Input: part model. Units: mm. Frame: model coordinates. A direction names the side the tool comes from. Coordinates: 2 decimals unless noted, no trailing zeros. Order: outer loops, then holes, each group sorted by start corner. A loop starts at its lowest first (then second) coordinate and runs counter-clockwise, first axis right, second up. Notation, with made-up numbers: (-6.75, 42) -> (35.25, 42) arc R25 cw to (35.25, 63) -> close; hole circle Ø1 at (-30, 3). An arc over 180 degrees is marked (long way). One line per question, with ' | ' between items.
```python
from build123d import *

# Parameters (mm, degrees)
SKETCH1_W           = 14.40065461
SKETCH1_H           = 29
SKETCH1_W_2         = 14
SKETCH1_R           = 1.35
BOSS_EXTRUDE2_DEPTH = 2
SKETCH2_R           = 7.5
CUT_EXTRUDE1_DEPTH  = 2
SKETCH3_W           = 5.497638463
SKETCH3_H           = 5.570940309
SKETCH3_W_2         = 9.162730771
SKETCH3_H_2         = 3.811696001
SKETCH3_W_3         = 6.450562463
SKETCH3_H_3         = 6.157355078
SKETCH3_W_4         = 5.570940309
SKETCH3_H_4         = 4.544714463
SKETCH3_W_5         = 6.27821864
SKETCH3_H_5         = 3.656250045
SKETCH3_W_6         = 6.338006476
SKETCH3_H_6         = 4.174139377
BOSS_EXTRUDE3_DEPTH = 2
SKETCH4_R           = 1.6
CUT_EXTRUDE2_DEPTH  = 10
CHAMFER1_SIZE       = 1
SKETCH5_W           = 10.813263603
SKETCH5_H           = 2.270321327
SKETCH5_W_2         = 10.386812418
SKETCH5_H_2         = 2.583327919
SKETCH5_W_3         = 10.884553744
SKETCH5_H_3         = 2.62287776
SKETCH5_W_4         = 12.051602383
SKETCH5_H_4         = 3.322696714
BOSS_EXTRUDE4_DEPTH = 2


with BuildPart() as part:
    # Sketch1 → Boss-Extrude2 (new body)
    with BuildSketch(Plane(origin=(0, 0, 0), x_dir=(1, 0, 0), z_dir=(0, 1, 0))):
        with Locations((-22.106428168, 0.106069008)):
            Rectangle(SKETCH1_W, SKETCH1_H)
        with Locations((21.693244527, 0.106069008)):
            Rectangle(SKETCH1_W_2, SKETCH1_H)
        with BuildLine():
            Line((22.693244527, -34.393930992), (26.693244527, -34.393930992))
            ThreePointArc((26.693244527, -34.393930992), (28.814564871, -33.515251336), (29.693244527, -31.393930992))
            Line((29.693244527, -31.393930992), (29.693244527, -24.393930992))
            Line((29.693244527, -24.393930992), (28.693244527, -24.393930992))
            Line((28.693244527, -24.393930992), (28.693244527, -14.393930992))
            Line((28.693244527, -14.393930992), (11.693244527, -14.393930992))
            Line((11.693244527, -14.393930992), (11.693244527, -26.393930992))
            Line((11.693244527, -26.393930992), (-12.306755473, -26.393930992))
            Line((-12.306755473, -26.393930992), (-12.306755473, -14.393930992))
            Line((-12.306755473, -14.393930992), (-29.306755473, -14.393930992))
            Line((-29.306755473, -14.393930992), (-29.306755473, -24.393930992))
            Line((-29.306755473, -24.393930992), (-30.306755473, -24.393930992))
            Line((-30.306755473, -24.393930992), (-30.306755473, -31.393930992))
            ThreePointArc((-30.306755473, -31.393930992), (-29.428075817, -33.515251336), (-27.306755473, -34.393930992))
            Line((-27.306755473, -34.393930992), (-25.306755473, -34.393930992))
            Line((-25.306755473, -34.393930992), (-25.306755473, -32.393930992))
            Line((-25.306755473, -32.393930992), (-15.306755473, -32.393930992))
            Line((-15.306755473, -32.393930992), (-15.306755473, -34.393930992))
            Line((-15.306755473, -34.393930992), (12.693244527, -34.393930992))
            Line((12.693244527, -34.393930992), (12.693244527, -32.393930992))
            Line((12.693244527, -32.393930992), (22.693244527, -32.393930992))
            Line((22.693244527, -32.393930992), (22.693244527, -34.393930992))
        make_face()
        with Locations((-20.98250428, -22.393930992)):
            Circle(SKETCH1_R, mode=Mode.SUBTRACT)
        with Locations((19.975772563, -22.393930992)):
            Circle(SKETCH1_R, mode=Mode.SUBTRACT)
        with Locations((-0.212217338, -28.393930992)):
            Circle(SKETCH1_R, mode=Mode.SUBTRACT)
        with BuildLine():
            Line((-23.306755473, 34.606069008), (-27.306755473, 34.606069008))
            ThreePointArc((-27.306755473, 34.606069008), (-29.428075817, 33.727389352), (-30.306755473, 31.606069008))
            Line((-30.306755473, 31.606069008), (-30.306755473, 24.606069008))
            Line((-30.306755473, 24.606069008), (-29.306755473, 24.606069008))
            Line((-29.306755473, 24.606069008), (-29.306755473, 14.606069008))
            Line((-29.306755473, 14.606069008), (28.693244527, 14.606069008))
            Line((28.693244527, 14.606069008), (28.693244527, 24.606069008))
            Line((28.693244527, 24.606069008), (29.693244527, 24.606069008))
            Line((29.693244527, 24.606069008), (29.693244527, 31.606069008))
            ThreePointArc((29.693244527, 31.606069008), (28.814564871, 33.727389352), (26.693244527, 34.606069008))
            Line((26.693244527, 34.606069008), (24.693244527, 34.606069008))
            Line((24.693244527, 34.606069008), (24.693244527, 32.606069008))
            Line((24.693244527, 32.606069008), (14.693244527, 32.606069008))
            Line((14.693244527, 32.606069008), (14.693244527, 34.606069008))
            Line((14.693244527, 34.606069008), (-13.306755473, 34.606069008))
            Line((-13.306755473, 34.606069008), (-13.306755473, 32.606069008))
            Line((-13.306755473, 32.606069008), (-23.306755473, 32.606069008))
            Line((-23.306755473, 32.606069008), (-23.306755473, 34.606069008))
        make_face()
        with Locations((-20.98250428, 22.606069008)):
            Circle(SKETCH1_R, mode=Mode.SUBTRACT)
        with Locations((-0.212217338, 28.606069008)):
            Circle(SKETCH1_R, mode=Mode.SUBTRACT)
        with Locations((19.975772563, 22.606069008)):
            Circle(SKETCH1_R, mode=Mode.SUBTRACT)
        with Locations((-0.212217338, 17.606069008)):
            Circle(SKETCH1_R, mode=Mode.SUBTRACT)
    extrude(amount=BOSS_EXTRUDE2_DEPTH)

    # Sketch2 → Cut-Extrude1 (cut)
    with BuildSketch(Plane(origin=(0, 2, 0), x_dir=(1, 0, 0), z_dir=(0, 1, 0))):
        with Locations((-0.212217338, 17.606069008)):
            Circle(SKETCH2_R)
    extrude(amount=-CUT_EXTRUDE1_DEPTH, mode=Mode.SUBTRACT)

    # Sketch3 → Boss-Extrude3 (add)
    with BuildSketch(Plane(origin=(0, 2, 0), x_dir=(1, 0, 0), z_dir=(0, 1, 0))):
        with Locations((-20.684668709, 22.829641321)):
            Rectangle(SKETCH3_W, SKETCH3_H)
        with Locations((0.426262988, 28.40058163)):
            Rectangle(SKETCH3_W_2, SKETCH3_H_2)
        with Locations((19.594695763, 21.950019167)):
            Rectangle(SKETCH3_W_3, SKETCH3_H_3)
        with Locations((20.03450684, -21.664579305)):
            Rectangle(SKETCH3_W_4, SKETCH3_H_4)
        with Locations((-1.015993077, -28.583465841)):
            Rectangle(SKETCH3_W_5, SKETCH3_H_5)
        with Locations((-20.264484702, -22.364159865)):
            Rectangle(SKETCH3_W_6, SKETCH3_H_6)
    extrude(amount=-BOSS_EXTRUDE3_DEPTH)

    # Sketch4 → Cut-Extrude2 (cut)
    with BuildSketch(Plane(origin=(0, 2, 0), x_dir=(1, 0, 0), z_dir=(0, 1, 0))):
        with BuildLine():
            ThreePointArc((-8.093244527, -27.893930992), (-8.379691654, -26.980378119), (-9.136468091, -26.393930992))
            Line((-9.136468091, -26.393930992), (-10.250020963, -26.393930992))
            ThreePointArc((-10.250020963, -26.393930992), (-10.6067974, -29.207483865), (-8.093244527, -27.893930992))
        make_face()
        with BuildLine():
            Line((-10.250020963, -26.393930992), (-9.136468091, -26.393930992))
            ThreePointArc((-9.136468091, -26.393930992), (-9.693244527, -26.293930992), (-10.250020963, -26.393930992))
        make_face()
        with Locations((-25.693244527, -27.893930992)):
            Circle(SKETCH4_R)
        with BuildLine():
            ThreePointArc((9.136468091, -26.393930992), (8.779691654, -29.207483865), (11.293244527, -27.893930992))
            ThreePointArc((11.293244527, -27.893930992), (11.0067974, -26.980378119), (10.250020963, -26.393930992))
            Line((10.250020963, -26.393930992), (9.136468091, -26.393930992))
        make_face()
        with BuildLine():
            Line((9.136468091, -26.393930992), (10.250020963, -26.393930992))
            ThreePointArc((10.250020963, -26.393930992), (9.693244527, -26.293930992), (9.136468091, -26.393930992))
        make_face()
        with Locations((25.693244527, -27.893930992)):
            Circle(SKETCH4_R)
        with Locations((25.693244527, 28.106069008)):
            Circle(SKETCH4_R)
        with Locations((9.693244527, 28.106069008)):
            Circle(SKETCH4_R)
        with Locations((-9.693244527, 28.106069008)):
            Circle(SKETCH4_R)
        with Locations((-25.693244527, 28.106069008)):
            Circle(SKETCH4_R)
    extrude(amount=-CUT_EXTRUDE2_DEPTH, mode=Mode.SUBTRACT)

    # Chamfer1
    chamfer1_edges = [part.edges().sort_by_distance(p)[0] for p in [
        (-27.293244527, 2, 27.893930992),
        (8.779691654, 2, 29.207483865),
        (24.093244527, 2, 27.893930992),
        (24.093244527, 2, -28.106069008),
        (8.093244527, 2, -28.106069008),
        (-11.293244527, 2, -28.106069008),
        (-27.293244527, 2, -28.106069008),
        (-10.6067974, 2, 29.207483865),
    ]]
    chamfer(chamfer1_edges, length=CHAMFER1_SIZE)

    # Sketch5 → Boss-Extrude4 (add)
    with BuildSketch(Plane(origin=(0, 2, 0), x_dir=(1, 0, 0), z_dir=(0, 1, 0))):
        with Locations((20.099876329, 33.470908345)):
            Rectangle(SKETCH5_W, SKETCH5_H)
        with Locations((-18.113349264, 33.314405048)):
            Rectangle(SKETCH5_W_2, SKETCH5_H_2)
        with Locations((-20.749032345, -33.082492112)):
            Rectangle(SKETCH5_W_3, SKETCH5_H_3)
        with Locations((16.667443335, -32.732582635)):
            Rectangle(SKETCH5_W_4, SKETCH5_H_4)
    extrude(amount=-BOSS_EXTRUDE4_DEPTH)


solid = part.part
```
1. Cut plane C-C, the plane y = 1.35. State how many separate pieces and enclosed holes the cut face has, and give its area (3 significant figures).
Recorded:
separate pieces: 1 | enclosed holes: 7 | area: 2,660 mm^2
2. Cut plane B-B, the plane x = -2. Return loops of the section in (y, z), and give its area (3 significant figures).
Recorded:
outline: (0, -34.61) -> (2, -34.61) -> (2, -24.89) -> (0, -24.89) -> close; (0, 26.39) -> (2, 26.39) -> (2, 34.39) -> (0, 34.39) -> close | area: 35.4 mm^2
3. Mould query, pull axis X, two halves, no side actions, for faces 5 (the face through (0, 1, 26.394)), 6 (the face through (-24.17, 0.51, -28.59)), 7 (the face through (28.79, 0.99, 33.54)), 8 (the face through (-29.451, 0.986, 33.492)). Classes: released by +X, released by -X, zero draft, split by the parting line, or undercut.
Recorded:
face 5: undercut | face 6: undercut | face 7: released by +X | face 8: released by -X
4. Ray query, line 1 (X direction, y = 0.9, z = 28); line 2 (Z direction, x = -0.5, y = 1.1); line 3 (X direction, y = 0.85, z = 25). Return the intervals inside material, ascending. Write a range as [from, to].
Recorded:
line 1: x = [-30.31, -27.29], [-24.1, -11.29], [-8.1, 8.1], [11.29, 24.1], [27.29, 29.69] | line 2: z = [-34.61, -25.1], [26.39, 34.39] | line 3: x = [-30.31, -12.31], [11.69, 29.69]
5. Cut plane A-A, the plane z = -12. Return loops of the section in (x, y), and give its area (3 significant figures).
Recorded:
outline: (-29.31, 0) -> (-14.91, 0) -> (-14.91, 2) -> (-29.31, 2) -> close; (14.69, 0) -> (28.69, 0) -> (28.69, 2) -> (14.69, 2) -> close | area: 56.8 mm^2
6. Access query for faces 1 (the face through (-11, 1, 26.394)), 2 (the face through (-29.307, 1, 0)), 3 (the face through (28.693, 1, 0)), 4 (the face through (-30.307, 1, -28)). Directions: +Z, -Z, +X, -X, +Y, -Y. A direction counts if a zero-diameter tool reaches every point of the face in a straight line with its end or side. Return the directions, or none.
Recorded:
face 1: +Y, -Y | face 2: -X, +Y, -Y | face 3: +X, +Y, -Y | face 4: +Z, -Z, -X, +Y, -Y
7. Pin query (flat end, axial travel): pin 1 Ø4 at (x, z) = (-9.69, -28.11) entering from +Y; pin 2 Ø1.1 at (x, y) = (29, 0.5) entering from +Z; pin 3 Ø1 at (y, z) = (1, 1) entering from +X; pin 4 Ø3 at (x, z) = (-25.69, 27.89) entering from +Y. Return the tip coordinate at first contact, or that it passes through.
Recorded:
pin 1: stops at y = 1.41 | pin 2: stops at z = 33.83 | pin 3: stops at x = 28.69 | pin 4: passes through
